```python
from build123d import *

# Parameters (mm, degrees)
SKETCH1_W               = 59
SKETCH1_H               = 50
BASE_FLANGE1_DEPTH      = 2
EDGE_FLANGE1_DEPTH      = 35
EDGE_FLANGE1_BEND_DEPTH = 35
EDGE_FLANGE2_DEPTH      = 31
EDGE_FLANGE2_BEND_DEPTH = 31
CUT_EXTRUDE1_REACH      = 69.359
CUT_EXTRUDE2_REACH      = 74.168
SKETCH19_R              = 2.55
CUT_EXTRUDE3_REACH      = 69.359
SKETCH20_R              = 7
BREAK_CORNER1_START     = -13
BREAK_CORNER1_DEPTH     = 2
BREAK_CORNER1_START_2   = -32.5
BREAK_CORNER1_2_DEPTH   = 65
BREAK_CORNER1_START_3   = -2
BREAK_CORNER1_3_DEPTH   = 2
CUT_EXTRUDE4_DEPTH      = 95.899947313


# Read off the part's stored shape, not the designer's step: Break-Corner1
# Sheet-metal steps are written as plain solids
with BuildPart() as part:
    # Sketch1 → Base-Flange1 (new body)
    with BuildSketch(Plane.XY):
        Rectangle(SKETCH1_W, SKETCH1_H)
    extrude(amount=-BASE_FLANGE1_DEPTH)

    # Edge-Flange1 section (across the edge) → Edge-Flange1 (add)
    with BuildSketch(Plane(origin=(30.5, 25, -2), x_dir=(-1, 0, 0), z_dir=(0, -1, 0))):
        with BuildLine():
            Line((-2, 1), (-2, 32))
            Line((-2, 32), (0, 32))
            Line((0, 32), (0, 1))
            ThreePointArc((0, 1), (0.292893219, 0.292893219), (1, 0))
            Line((1, 0), (1, -2))
            ThreePointArc((1, -2), (-1.121320344, -1.121320344), (-2, 1))
        make_face()
    extrude(amount=EDGE_FLANGE1_DEPTH)

    # Edge-Flange1 section 2 (across the edge) → Edge-Flange1 bend (add)
    with BuildSketch(Plane(origin=(-30.5, -10, -2), x_dir=(1, 0, 0), z_dir=(0, 1, 0))):
        with BuildLine():
            Line((-2, 1), (-2, 32))
            Line((-2, 32), (0, 32))
            Line((0, 32), (0, 1))
            ThreePointArc((0, 1), (0.292893219, 0.292893219), (1, 0))
            Line((1, 0), (1, -2))
            ThreePointArc((1, -2), (-1.121320344, -1.121320344), (-2, 1))
        make_face()
    extrude(amount=EDGE_FLANGE1_BEND_DEPTH)

    # Edge-Flange2 section (across the edge) → Edge-Flange2 (add)
    with BuildSketch(Plane(origin=(32.5, -11, -3), x_dir=(0, 1, 0), z_dir=(0, 0, -1))):
        with BuildLine():
            Line((-2, 1), (-2, 20))
            Line((-2, 20), (0, 20))
            Line((0, 20), (0, 1))
            ThreePointArc((0, 1), (0.292893219, 0.292893219), (1, 0))
            Line((1, 0), (1, -2))
            ThreePointArc((1, -2), (-1.121320344, -1.121320344), (-2, 1))
        make_face()
    extrude(amount=EDGE_FLANGE2_DEPTH)

    # Edge-Flange2 section 2 (across the edge) → Edge-Flange2 bend (add)
    with BuildSketch(Plane(origin=(-32.5, -11, -34), x_dir=(0, 1, 0), z_dir=(0, 0, 1))):
        with BuildLine():
            Line((-2, 1), (-2, 20))
            Line((-2, 20), (0, 20))
            Line((0, 20), (0, 1))
            ThreePointArc((0, 1), (0.292893219, 0.292893219), (1, 0))
            Line((1, 0), (1, -2))
            ThreePointArc((1, -2), (-1.121320344, -1.121320344), (-2, 1))
        make_face()
    extrude(amount=EDGE_FLANGE2_BEND_DEPTH)

    # Sketch18 → Cut-Extrude1 (cut, up to next)
    with BuildSketch(Plane.XY, mode=Mode.PRIVATE) as cut_extrude1_sk1:
        with BuildLine():
            Line((-20.95, 2.5), (-20.95, -17.5))
            ThreePointArc((-20.95, -17.5), (-23, -19.55), (-25.05, -17.5))
            Line((-25.05, -17.5), (-25.05, 2.5))
            ThreePointArc((-25.05, 2.5), (-23, 4.55), (-20.95, 2.5))
        make_face()
    cut_extrude1_tool1 = extrude(cut_extrude1_sk1.sketch, amount=-CUT_EXTRUDE1_REACH, mode=Mode.PRIVATE) & part.part
    # Sketch18 → Cut-Extrude1 (cut, up to next)
    with BuildSketch(Plane.XY, mode=Mode.PRIVATE) as cut_extrude1_sk2:
        with BuildLine():
            Line((20.95, -17.5), (20.95, 2.5))
            ThreePointArc((20.95, 2.5), (23, 4.55), (25.05, 2.5))
            Line((25.05, 2.5), (25.05, -17.5))
            ThreePointArc((25.05, -17.5), (23, -19.55), (20.95, -17.5))
        make_face()
    cut_extrude1_tool2 = extrude(cut_extrude1_sk2.sketch, amount=-CUT_EXTRUDE1_REACH, mode=Mode.PRIVATE) & part.part
    add(cut_extrude1_tool1.solids().sort_by_distance((-23, -7.5, 0))[0], mode=Mode.SUBTRACT)
    add(cut_extrude1_tool2.solids().sort_by_distance((23, -7.5, 0))[0], mode=Mode.SUBTRACT)

    # Sketch19 → Cut-Extrude2 (cut, up to next)
    with BuildSketch(Plane(origin=(0, -11, 0), x_dir=(1, 0, 0), z_dir=(0, 1, 0)), mode=Mode.PRIVATE) as cut_extrude2_sk1:
        with Locations(Location((43, 18.5, 0), (0, 0, 180))):
            Circle(SKETCH19_R)
    cut_extrude2_tool1 = extrude(cut_extrude2_sk1.sketch, amount=-CUT_EXTRUDE2_REACH, mode=Mode.PRIVATE) & part.part
    # Sketch19 → Cut-Extrude2 (cut, up to next)
    with BuildSketch(Plane(origin=(0, -11, 0), x_dir=(1, 0, 0), z_dir=(0, 1, 0)), mode=Mode.PRIVATE) as cut_extrude2_sk2:
        with Locations(Location((-43, 18.5, 0), (0, 0, 180))):
            Circle(SKETCH19_R)
    cut_extrude2_tool2 = extrude(cut_extrude2_sk2.sketch, amount=-CUT_EXTRUDE2_REACH, mode=Mode.PRIVATE) & part.part
    add(cut_extrude2_tool1.solids().sort_by_distance((43, -11, -18.5))[0], mode=Mode.SUBTRACT)
    add(cut_extrude2_tool2.solids().sort_by_distance((-43, -11, -18.5))[0], mode=Mode.SUBTRACT)

    # Sketch20 → Cut-Extrude3 (cut, up to next)
    with BuildSketch(Plane.XY, mode=Mode.PRIVATE) as cut_extrude3_sk1:
        Circle(SKETCH20_R)
    cut_extrude3_tool1 = extrude(cut_extrude3_sk1.sketch, amount=-CUT_EXTRUDE3_REACH, mode=Mode.PRIVATE) & part.part
    # Sketch20 → Cut-Extrude3 (cut, up to next)
    with BuildSketch(Plane.XY, mode=Mode.PRIVATE) as cut_extrude3_sk2:
        with BuildLine():
            ThreePointArc((-7, 0), (0, 7), (7, 0))
            Line((7, 0), (7, 25))
            Line((7, 25), (-7, 25))
            Line((-7, 25), (-7, 0))
        make_face()
    cut_extrude3_tool2 = extrude(cut_extrude3_sk2.sketch, amount=-CUT_EXTRUDE3_REACH, mode=Mode.PRIVATE) & part.part
    add(cut_extrude3_tool1.solids().sort_by_distance((0, 0, 0))[0], mode=Mode.SUBTRACT)
    add(cut_extrude3_tool2.solids().sort_by_distance((0, 15.186311, 0))[0], mode=Mode.SUBTRACT)

    # Break-Corner1 outline → Break-Corner1 (cut)
    with BuildSketch(Plane(origin=(0, 0, 0), x_dir=(1, 0, 0), z_dir=(0, 1, 0)).offset(BREAK_CORNER1_START)):
        with BuildLine():
            ThreePointArc((50.5, 34), (51.914213562, 33.414213562), (52.5, 32))
            Line((52.5, 32), (52.5, 34))
            Line((52.5, 34), (50.5, 34))
        make_face()
        with BuildLine():
            ThreePointArc((52.5, 5), (51.914213562, 3.585786438), (50.5, 3))
            Line((50.5, 3), (52.5, 3))
            Line((52.5, 3), (52.5, 5))
        make_face()
        with BuildLine():
            ThreePointArc((-50.5, 3), (-51.914213562, 3.585786438), (-52.5, 5))
            Line((-52.5, 5), (-52.5, 3))
            Line((-52.5, 3), (-50.5, 3))
        make_face()
        with BuildLine():
            ThreePointArc((-52.5, 32), (-51.914213562, 33.414213562), (-50.5, 34))
            Line((-50.5, 34), (-52.5, 34))
            Line((-52.5, 34), (-52.5, 32))
        make_face()
    extrude(amount=BREAK_CORNER1_DEPTH, mode=Mode.SUBTRACT)

    # Break-Corner1 2 outline → Break-Corner1 2 (cut)
    with BuildSketch(Plane.YZ.offset(BREAK_CORNER1_START_2)):
        with BuildLine():
            Line((25, -34), (25, -32))
            ThreePointArc((25, -32), (24.414213562, -33.414213562), (23, -34))
            Line((23, -34), (25, -34))
        make_face()
    extrude(amount=BREAK_CORNER1_2_DEPTH, mode=Mode.SUBTRACT)

    # Break-Corner1 3 outline → Break-Corner1 3 (cut)
    with BuildSketch(Plane.XY.offset(BREAK_CORNER1_START_3)):
        with BuildLine():
            Line((7, 25), (7, 23))
            ThreePointArc((7, 23), (7.585786438, 24.414213562), (9, 25))
            Line((9, 25), (7, 25))
        make_face()
        with BuildLine():
            Line((-29.5, -25), (-27.5, -25))
            ThreePointArc((-27.5, -25), (-28.914213562, -24.414213562), (-29.5, -23))
            Line((-29.5, -23), (-29.5, -25))
        make_face()
        with BuildLine():
            ThreePointArc((29.5, -23), (28.914213562, -24.414213562), (27.5, -25))
            Line((27.5, -25), (29.5, -25))
            Line((29.5, -25), (29.5, -23))
        make_face()
        with BuildLine():
            ThreePointArc((-9, 25), (-7.585786438, 24.414213562), (-7, 23))
            Line((-7, 23), (-7, 25))
            Line((-7, 25), (-9, 25))
        make_face()
    extrude(amount=BREAK_CORNER1_3_DEPTH, mode=Mode.SUBTRACT)

    # Sketch21 → Cut-Extrude4 (cut, through all)
    with BuildSketch(Plane.ZY.offset(32.5)):
        with BuildLine():
            Line((-21.616666667, 15), (-21.616666667, 0))
            ThreePointArc((-21.616666667, 0), (-23.666666667, -2.05), (-25.716666667, 0))
            Line((-25.716666667, 0), (-25.716666667, 15))
            ThreePointArc((-25.716666667, 15), (-23.666666667, 17.05), (-21.616666667, 15))
        make_face()
        with BuildLine():
            Line((-11.283333333, 15), (-11.283333333, 0))
            ThreePointArc((-11.283333333, 0), (-13.333333333, -2.05), (-15.383333333, 0))
            Line((-15.383333333, 0), (-15.383333333, 15))
            ThreePointArc((-15.383333333, 15), (-13.333333333, 17.05), (-11.283333333, 15))
        make_face()
    extrude(amount=-CUT_EXTRUDE4_DEPTH, mode=Mode.SUBTRACT)


solid = part.part
```
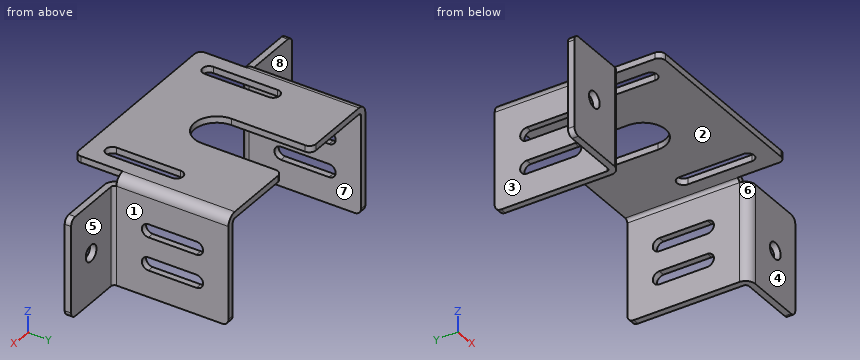
Geometry check sheet. Reference: the model listing, model coordinates, mm. Face numbers are marked on the shaded views. A direction names the side the tool comes from. Round coordinates to 2 decimals unless told otherwise and drop trailing zeros. Order: outer loops, then holes, each group sorted by start corner. A loop starts at its lowest first (then second) coordinate and runs counter-clockwise, first axis right, second up. Notation, with made-up numbers: (-34.75, 22.25) -> (-21.75, 22.25) arc R20 ccw to (-21.75, 38.25) -> close; hole circle Ø6 at (74.5, 25.25). An arc over 180 degrees is marked (long way). Return JSON: item names as keys, results as strings. Group by question number.
Q1. Section check D-D, the plane x = -23. Record the boundary of the cut face in (y, z).
Q2. Tool access check on the marked faces 4, 5, 6, 7 and 8. Record the directions out of +Z, -Z, +X, -X, +Y, -Y that give a thin tool (end or side, any length) a straight path to the whole face; none if there is none.
Q3. Section check C-C, the plane z = -18.5. Record the boundary of the cut face in (x, y), plus the area to 3 significant figures.
Q4. Release check for a two-part mould opening along X. For the marked faces 1, 2 and 3 record: released by +X, released by -X, zero draft, split by the parting line, or undercut.
Q5. Gauge pin test, flat ends, axial feed: pin 1 (6 mm diameter, centred on x = -43, z = -18.5, fed in from +Y); pin 2 (9.5 mm diameter, centred on y = 8, z = -17, fed in from -X); pin 3 (2 mm diameter, centred on y = 16, z = -8.5, fed in from +X). Record the tip position at first contact, or that the pin passes through.
Q6. Section check B-B, the plane y = -14.5. Record the boundary of the cut face in (x, z), plus the area to 3 significant figures.
Q7. Material ranges on probe 1 along Z at (x, y) = (-43, -12.35); probe 2 along X at (y, z) = (-8, -26.5); probe 3 along X at (y, z) = (-12, -18), recorded low to high. Write a range as from..to.
Q8. Section check A-A, the plane z = -6.5. Record the boundary of the cut face in (x, y), plus the area to 3 significant figures.
Numbers:
{
 "1": {"outline": "(-25, -2) -> (-19.55, -2) -> (-19.55, 0) -> (-25, 0) -> close; (4.55, -2) -> (25, -2) -> (25, 0) -> (4.55, 0) -> close"},
 "2": {"face 4": "+Z, -Z, +X, -X, -Y", "face 5": "+Z, -Z, +X, +Y", "face 6": "+Z, -Z, -Y", "face 7": "-Z, +Y, -Y", "face 8": "+Z, -Z, -X, +Y"},
 "3": {"outline": "(-52.5, -13) -> (-45.55, -13) -> (-45.55, -11) -> (-52.5, -11) -> close; (-40.45, -13) -> (-33.5, -13) arc R3 ccw to (-30.5, -10) -> (-30.5, 25) -> (-32.5, 25) -> (-32.5, -10) arc R1 cw to (-33.5, -11) -> (-40.45, -11) -> close; (30.5, -10) arc R3 ccw to (33.5, -13) -> (40.45, -13) -> (40.45, -11) -> (33.5, -11) arc R1 cw to (32.5, -10) -> (32.5, 25) -> (30.5, 25) -> close; (45.55, -13) -> (52.5, -13) -> (52.5, -11) -> (45.55, -11) -> close", "area": "208 mm^2"},
 "4": {"face 1": "released by +X", "face 2": "undercut", "face 3": "released by -X"},
 "5": {"pin 1": "y = -11", "pin 2": "x = -32.5", "pin 3": "x = 32.5"},
 "6": {"outline": "(-29.5, -2) -> (-25.05, -2) -> (-25.05, 0) -> (-29.5, 0) -> close; (-20.95, -2) -> (20.95, -2) -> (20.95, 0) -> (-20.95, 0) -> close; (25.05, -2) -> (29.5, -2) -> (29.5, 0) -> (25.05, 0) -> close", "area": "102 mm^2"},
 "7": {"probe 1": "-34..-21.05, -15.95..-3", "probe 2": "-32.5..-30.5, 30.5..32.5", "probe 3": "-52.5..-45.5, -40.5..-31.26, 31.26..40.5, 45.5..52.5"},
 "8": {"outline": "(-52.5, -13) -> (-33.5, -13) arc R3 ccw to (-30.5, -10) -> (-30.5, 25) -> (-32.5, 25) -> (-32.5, -10) arc R1 cw to (-33.5, -11) -> (-52.5, -11) -> close; (30.5, -10) arc R3 ccw to (33.5, -13) -> (52.5, -13) -> (52.5, -11) -> (33.5, -11) arc R1 cw to (32.5, -10) -> (32.5, 25) -> (30.5, 25) -> close", "area": "229 mm^2"}
}
